from build123d import *

# Parameters (mm, degrees)
SKETCH1_W           = 101.6
SKETCH1_H           = 82.55
BOSS_EXTRUDE1_DEPTH = 3.175
SKETCH2_W           = 101.6
SKETCH2_H           = 82.55
BOSS_EXTRUDE2_DEPTH = 3.175
FILLET1_R           = 0.9525
SKETCH3_W           = 12.7
SKETCH3_H           = 82.55
BOSS_EXTRUDE3_DEPTH = 9.525
SKETCH4_W           = 12.7
SKETCH4_H           = 82.55
BOSS_EXTRUDE4_DEPTH = 9.525
FILLET2_R           = 3.175
CUT_EXTRUDE2_DEPTH  = 111.396900432


with BuildPart() as part:
    # Sketch1 → Boss-Extrude1 (new body)
    with BuildSketch(Plane(origin=(0, 0, 0), x_dir=(0, 0, -1), z_dir=(1, 0, 0))):
        Rectangle(SKETCH1_W, SKETCH1_H)
    extrude(amount=BOSS_EXTRUDE1_DEPTH)

    # Sketch2 → Boss-Extrude2 (add)
    with BuildSketch(Plane(origin=(3.175, 0, 0), x_dir=(0, 0, -1), z_dir=(1, 0, 0))):
        Rectangle(SKETCH2_W, SKETCH2_H)
        with BuildLine():
            ThreePointArc((-40.340733258, 27.65848557), (-43.020329338, 27.945699456), (-44.45, 25.661236989))
            Line((-44.45, 25.661236989), (-44.45, -25.661236989))
            ThreePointArc((-44.45, -25.661236989), (-43.020329338, -27.945699456), (-40.340733258, -27.65848557))
            Line((-40.340733258, -27.65848557), (-7.68097709, -1.997248581))
            ThreePointArc((-7.68097709, -1.997248581), (-6.710243832, 0), (-7.68097709, 1.997248581))
            Line((-7.68097709, 1.997248581), (-40.340733258, 27.65848557))
        make_face(mode=Mode.SUBTRACT)
        with BuildLine():
            Line((33.536295637, -30.387751419), (1.569266742, -5.270800144))
            ThreePointArc((1.569266742, -5.270800144), (0, -4.728048725), (-1.569266742, -5.270800144))
            Line((-1.569266742, -5.270800144), (-33.536295637, -30.387751419))
            ThreePointArc((-33.536295637, -30.387751419), (-34.367509201, -33.215237498), (-31.967028895, -34.925))
            Line((-31.967028895, -34.925), (31.967028895, -34.925))
            ThreePointArc((31.967028895, -34.925), (34.367509201, -33.215237498), (33.536295637, -30.387751419))
        make_face(mode=Mode.SUBTRACT)
        with BuildLine():
            Line((40.340733258, 27.65848557), (7.68097709, 1.997248581))
            ThreePointArc((7.68097709, 1.997248581), (6.710243832, 0), (7.68097709, -1.997248581))
            Line((7.68097709, -1.997248581), (40.340733258, -27.65848557))
            ThreePointArc((40.340733258, -27.65848557), (43.020329338, -27.945699456), (44.45, -25.661236989))
            Line((44.45, -25.661236989), (44.45, 25.661236989))
            ThreePointArc((44.45, 25.661236989), (43.020329338, 27.945699456), (40.340733258, 27.65848557))
        make_face(mode=Mode.SUBTRACT)
        with BuildLine():
            Line((-33.536295637, 30.387751419), (-1.569266742, 5.270800144))
            ThreePointArc((-1.569266742, 5.270800144), (0, 4.728048725), (1.569266742, 5.270800144))
            Line((1.569266742, 5.270800144), (33.536295637, 30.387751419))
            ThreePointArc((33.536295637, 30.387751419), (34.367509201, 33.215237498), (31.967028895, 34.925))
            Line((31.967028895, 34.925), (-31.967028895, 34.925))
            ThreePointArc((-31.967028895, 34.925), (-34.367509201, 33.215237498), (-33.536295637, 30.387751419))
        make_face(mode=Mode.SUBTRACT)
    extrude(amount=BOSS_EXTRUDE2_DEPTH)

    # Fillet1
    fillet1_edges = [part.edges().sort_by_distance(p)[0] for p in [
        (3.175, 33.215237498, 34.367509201),
        (3.175, 17.829275782, -17.55278119),
        (3.175, 27.945699456, -43.020329338),
        (3.175, -33.215237498, -34.367509201),
        (3.175, -34.925, 0),
        (3.175, 0, 6.710243832),
        (3.175, -14.827867075, 24.010855174),
        (3.175, -27.945699456, 43.020329338),
        (3.175, 0, -6.710243832),
        (3.175, -4.728048725, 0),
        (3.175, 0, 44.45),
        (3.175, 4.728048725, 0),
        (3.175, 27.945699456, 43.020329338),
        (3.175, 14.827867075, 24.010855174),
        (3.175, -17.829275782, -17.55278119),
        (3.175, -17.829275782, 17.55278119),
        (3.175, -33.215237498, 34.367509201),
        (3.175, 14.827867075, -24.010855174),
        (3.175, -14.827867075, -24.010855174),
        (3.175, -27.945699456, -43.020329338),
        (3.175, 0, -44.45),
        (3.175, 17.829275782, 17.55278119),
        (3.175, 33.215237498, -34.367509201),
        (3.175, 34.925, 0),
    ]]
    fillet(fillet1_edges, radius=FILLET1_R)

    # Sketch3 → Boss-Extrude3 (add)
    with BuildSketch(Plane(origin=(0, 0, -50.8), x_dir=(-1, 0, 0), z_dir=(0, 0, -1))):
        with Locations((6.35, 0)):
            Rectangle(SKETCH3_W, SKETCH3_H)
    extrude(amount=-BOSS_EXTRUDE3_DEPTH)

    # Sketch4 → Boss-Extrude4 (add)
    with BuildSketch(Plane.XY.offset(50.8)):
        with Locations((-6.35, 0)):
            Rectangle(SKETCH4_W, SKETCH4_H)
    extrude(amount=-BOSS_EXTRUDE4_DEPTH)

    # Fillet2
    fillet2_edges = [part.edges().sort_by_distance(p)[0] for p in [
        (0, 0, 41.275),
        (0, 0, -41.275),
    ]]
    fillet(fillet2_edges, radius=FILLET2_R)

    # Sketch5 → Cut-Extrude2 (cut, through all)
    with BuildSketch(Plane.XY.offset(50.8)):
        with BuildLine():
            Line((-12.7, 29.36875), (-6.35, 29.36875))
            ThreePointArc((-6.35, 29.36875), (-3.96875, 31.75), (-6.35, 34.13125))
            Line((-6.35, 34.13125), (-12.7, 34.13125))
            Line((-12.7, 34.13125), (-12.7, 29.36875))
        make_face()
        with BuildLine():
            Line((-12.7, -34.13125), (-6.35, -34.13125))
            ThreePointArc((-6.35, -34.13125), (-3.96875, -31.75), (-6.35, -29.36875))
            Line((-6.35, -29.36875), (-12.7, -29.36875))
            Line((-12.7, -29.36875), (-12.7, -34.13125))
        make_face()
    extrude(amount=-CUT_EXTRUDE2_DEPTH, mode=Mode.SUBTRACT)


solid = part.part
Input: part model. Units: mm. Frame: model coordinates. A direction names the side the tool comes from. Coordinates: 2 decimals unless noted, no trailing zeros. Write item = value, one per line. Start each with the question number.
(1) First-contact query: P1, Ø8.5, axis at y = -25, z = 12, coming from the +X side (3 decimals); P2, Ø23, axis at y = -8.5, z = -16.5, coming from the -X side. Flat tips, straight axial feed; report the tip coordinate or a pass-through.
(2) Pull-direction query (Z, two-part tool) for faces 1 (the flat face through (3.175, 0, 30)), 2 (the flat face through (6.35, 1, 1)); classes: released by +Z, released by -Z, zero draft, split by the parting line, or undercut.
(3) Line query: line 1 along Y through (x, z) = (-7.5, -42) (3 decimals); line 2 along Z through (x, y) = (-8.5, -1) (3 decimals); line 3 along Z through (x, y) = (-1.75, -18). Output: solid intervals per line, ascending. Write a range as [from, to].
(4) Reachability of faces 3 (the cylindrical face through (5.22, 4.73, 0.02)), 4 (the flat face through (-9, 34.131, -46)), 5 (the flat face through (-8, 1, -41.275)) from +Z, -Z, +X, -X, +Y, -Y: full face, straight path, thin tool, end or side. Return the list, or none.
Result set:
q1.P1 = 3.175
q1.P2 = 0
q2.face_1 = undercut
q2.face_2 = zero draft
q3.line_1 = [-41.275, -34.131], [-29.369, 29.369], [34.131, 41.275]
q3.line_2 = [-50.8, -41.275], [41.275, 50.8]
q3.line_3 = [-50.8, -40.94], [40.94, 50.8]
q4.face_3 = +X
q4.face_4 = +Z, -Z, -X
q4.face_5 = -X, +Y, -Y
